Read the model definition and answer for the solid it produces. Units are mm, in the model's axes. Face numbers are marked on the shaded views. A direction names the side the tool comes from. Coordinates: 2 decimals unless noted, no trailing zeros. Write each loop counter-clockwise with the first axis right and the second up, starting at its lowest first coordinate (ties: lowest second). Pieces come first, ordered by that corner, then holes. Notation, with made-up numbers: (52, -18) - (80, -18) arc R14 cw to (80, -9) - close; hole circle Ø10 at (26, 47.25). An arc over 180 degrees is marked (long way). Use a Markdown table: item, result.
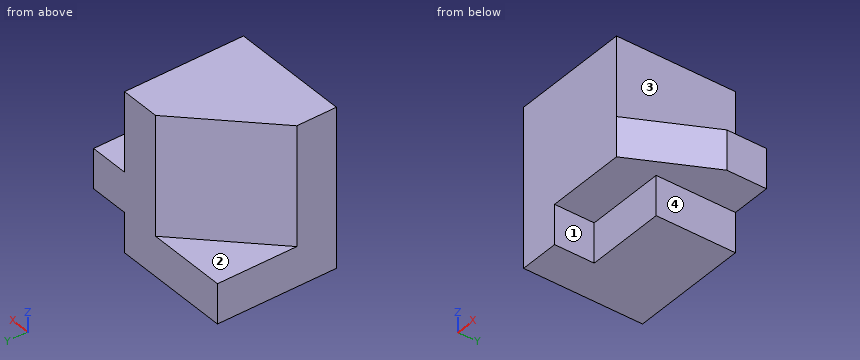
from build123d import *

# Parameters (mm, degrees)
F0_W      = 40
F0_H      = 40
F1_DEPTH  = 30
F2_W      = 10
F2_H      = 20
F2_H_2    = 10
F3_DEPTH  = 30
F4_W      = 20
F4_H      = 10
F5_DEPTH  = 10
F7_DEPTH  = 10
F9_DEPTH  = 30
F10_ANGLE = 90


with BuildPart() as f1:
    # F0 (on Top) → F1 (new body)
    with BuildSketch(Plane.XY):
        Rectangle(F0_W, F0_H)
    extrude(amount=F1_DEPTH)

    # F2 (on face) → F3 (cut)
    with BuildSketch(Plane.XY.offset(30)):
        with Locations((15, 10)):
            Rectangle(F2_W, F2_H)
        with Locations((15, -15)):
            Rectangle(F2_W, F2_H_2)
    extrude(amount=-F3_DEPTH, mode=Mode.SUBTRACT)

    # F4 (on face) → F5 (cut)
    with BuildSketch(Plane.XZ.offset(20)):
        with Locations((0, 25)):
            Rectangle(F4_W, F4_H)
    extrude(amount=-F5_DEPTH, mode=Mode.SUBTRACT)

    # F6 (on face) → F7 (cut)
    with BuildSketch(Plane.XZ.offset(10)):
        Polygon((20, 10), (20, 30), (10, 30), align=None)
    extrude(amount=-F7_DEPTH, mode=Mode.SUBTRACT)

    # F8 (on face) → F9 (cut)
    with BuildSketch(Plane(origin=(0, 20, 0), x_dir=(-1, 0, 0), z_dir=(0, 1, 0))):
        Polygon((0, 0), (20, 0), (20, 20), align=None)
    extrude(amount=-F9_DEPTH, mode=Mode.SUBTRACT)


with BuildPart() as f1_1:
    # F10: moved
    add(f1.part.rotate(Axis((-5, -20, 0), (1, 0, 0)), F10_ANGLE))


solid = f1_1.part
(1) A cutting plane is placed at C-C, the plane z = 36. Write down the section's boundary in (x, y), and give its area (3 significant figures).
Report:
| item | result |
|---|---|
| outline | (-20, -50) - (10, -50) - (10, -20) - (0, -20) - (-20, -40) - close |
| area | 700 mm² |
(2) A cutting plane is placed at B-B, the plane x = -1.5. Write down the section's boundary in (y, z).
Report:
| item | result |
|---|---|
| outline | (-50, 10) - (-40, 10) - (-40, 0) - (-20, 0) - (-20, 10) - (-21.5, 10) - (-21.5, 40) - (-50, 40) - close |
(3) For the marked faces 1, 2, 3 and 4, determine the directions among +Z, -Z, +X, -X, +Y, -Y from which every point of the face is accessible in a straight line to the end or side of a thin tool.
Report:
| item | result |
|---|---|
| face 1 | -Z, +X, -Y |
| face 2 | +Z, -X, +Y |
| face 3 | +Z, +X, +Y, -Y |
| face 4 | -Z, +X, +Y, -Y |
(4) A cutting plane is placed at D-D, the plane y = -29. Write down the section's boundary in (x, z).
Report:
| item | result |
|---|---|
| outline | (-20, 0) - (10, 0) - (10, 10) - (20, 10) - (20, 20) - (10, 20) - (10, 40) - (-9, 40) - (-9, 10) - (-20, 10) - close |
(5) A cutting plane is placed at A-A, the plane y = -45. Write down the section's boundary in (x, z).
Report:
| item | result |
|---|---|
| outline | (-20, 0) - (-10, 0) - (-10, 10) - (12.5, 10) - (12.5, 20) - (10, 20) - (10, 40) - (-20, 40) - close |
(6) Straight lines are drawn through the part: L1, parallel to Z at x = 16, y = -36; L2, parallel to X at y = -33.5, z = 4; L3, parallel to Z at x = -8, y = -24.5. For each, find the intervals that lie inside material, in ascending order.
Report:
| item | result |
|---|---|
| L1 | z = 10 to 20 |
| L2 | x = -20 to 10 |
| L3 | z = 0 to 10 |
(7) Each of these flat-tipped pins is pushed along its axis until it touches: P1, Ø3, axis at y = -26.5, z = 5.5, coming from the +X side; P2, Ø8, axis at x = 16, y = -35.5, coming from the +Z side; P3, Ø4, axis at x = -14, z = 27, coming from the +Y side; P4, Ø12, axis at x = 11.5, z = 7.5, coming from the +Y side. Where does it stop, or does it pass through?
Report:
| item | result |
|---|---|
| P1 | stops at x = 10 |
| P2 | stops at z = 20 |
| P3 | stops at y = -32 |
| P4 | stops at y = -20 |
